```python
from build123d import *

# Parameters (mm, degrees)
SKETCH_2_W          = 51.075539497
SKETCH_2_H          = 30.123383878
CUT_EXTRUDE_1_DEPTH = 40
SKETCH_3_W          = 2.341501377
SKETCH_3_H          = 8.048910983
SKETCH_3_W_2        = 1.756126033
SKETCH_3_H_2        = 6.841574336
CUT_EXTRUDE_2_DEPTH = 20


with BuildPart() as part:
    # Эскиз1 → Повернуть1 (revolve)
    with BuildSketch(Plane.XY, mode=Mode.PRIVATE) as revolve_1_sk:
        Polygon((-9.75, 20), (-8.75, 20), (-8.75, 11), (8.75, 11), (8.75, 20), (9.75, 20), (9.75, 10), (-9.75, 10), align=None)
    revolve(revolve_1_sk.sketch.rotate(Axis((-17.336723769, 0, 0), (1, 0, 0)), 90), axis=Axis((-17.336723769, 0, 0), (1, 0, 0)))

    # Эскиз2 → Вырез-Вытянуть1 (cut)
    with BuildSketch(Plane(origin=(9.75, 0, 0), x_dir=(0, 0, -1), z_dir=(1, 0, 0))):
        with Locations((-1.37941238, -13.061691939)):
            Rectangle(SKETCH_2_W, SKETCH_2_H)
    extrude(amount=-CUT_EXTRUDE_1_DEPTH, mode=Mode.SUBTRACT)

    # Эскиз3 → Вырез-Вытянуть2 (cut)
    with BuildSketch(Plane(origin=(9.75, 0, 0), x_dir=(0, 0, -1), z_dir=(1, 0, 0))):
        with Locations((-20.670750689, 2.548643467)):
            Rectangle(SKETCH_3_W, SKETCH_3_H)
        with Locations((20.378063017, 2.310834734)):
            Rectangle(SKETCH_3_W_2, SKETCH_3_H_2)
    extrude(amount=-CUT_EXTRUDE_2_DEPTH, mode=Mode.SUBTRACT)


solid = part.part
```
Read the model definition and answer for the solid it produces. Units are mm, in the model's axes. A direction names the side the tool comes from. Give positions to 0.01 mm unless a question says otherwise; leave off trailing zeros. Order: outer loops, then holes, each group sorted by start corner. A loop starts at its lowest first (then second) coordinate and runs counter-clockwise, first axis right, second up. Notation, with made-up numbers: (-36, 6.5) -> (-23, 6.5) arc R24 cw to (-23, 17.5) -> close; hole circle Ø5 at (31.5, -28.75). An arc over 180 degrees is marked (long way). Write item = value, one per line.
1. A cutting plane is placed at B-B, the plane z = 14. Write down the section's boundary in (x, y), and give its area (3 significant figures).
Numbers:
outline = (-9.75, 2) -> (-8.75, 2) -> (-8.75, 14.28) -> (-9.75, 14.28) -> close; (8.75, 2) -> (9.75, 2) -> (9.75, 14.28) -> (8.75, 14.28) -> close
area = 24.6 mm²
2. A cutting plane is placed at A-A, the plane y = 12. Write down the section's boundary in (x, z).
Numbers:
outline = (-9.75, -16) -> (-8.75, -16) -> (-8.75, 16) -> (-9.75, 16) -> close; (8.75, -16) -> (9.75, -16) -> (9.75, 16) -> (8.75, 16) -> close
3. The mould has two halves that part along X. Classify faces 1 (the face through (0, 11, 0)), 2 (the face through (9.75, 11, 0)), 3 (the face through (9, 3, 19.5)), 4 (the face through (-9.75, 11, 0)): +X half, -X half, draft (parallel to the pull), parting line (faces both ways), or undercut.
Numbers:
face_1 = undercut
face_2 = +X half
face_3 = draft
face_4 = -X half
4. For faces 5 (the face through (-9, 3, 19.5)), 6 (the face through (8.75, 13, 0)), determine the directions among +Z, -Z, +X, -X, +Y, -Y from which every point of the face is accessible in a straight line to the end or side of a thin tool.
Numbers:
face_5 = +Z, +X, -X, +Y, -Y
face_6 = +Y
5. Given pin 1 (1.5 mm diameter, centred on x = -1.5, z = 4, fed in from -Y); pin 2 (2 mm diameter, centred on x = -7, z = 3.5, fed in from +Y); pin 3 (8 mm diameter, centred on x = 4, z = -4, fed in from -Y), each flat-ended and moving along its own axis, determine where each tip first touches the part or whether it passes through.
Numbers:
pin_1 = 8.8
pin_2 = 10.71
pin_3 = 6
6. Straight lines are drawn through the part: line 1 along X through (y, z) = (14, 5); line 2 along Z through (x, y) = (5.5, 8.5); line 3 along Z through (x, y) = (-1.25, 4). For each, find the intervals that lie inside material, in ascending order.
Numbers:
line_1 = -9.75 to -8.75, 8.75 to 9.75
line_2 = -6.98 to -5.27, 5.27 to 6.98
line_3 = -10.25 to -9.17, 9.17 to 10.25
7. A cutting plane is placed at D-D, the plane z = 8. Write down the section's boundary in (x, y), and give its area (3 significant figures).
Numbers:
outline = (-9.75, 6) -> (9.75, 6) -> (9.75, 18.33) -> (8.75, 18.33) -> (8.75, 7.55) -> (-8.75, 7.55) -> (-8.75, 18.33) -> (-9.75, 18.33) -> close
area = 51.8 mm²
8. A cutting plane is placed at C-C, the plane x = -1.5. Write down the section's boundary in (y, z).
Numbers:
outline = (2, -10.82) arc R11 ccw to (2, 10.82) -> (2, 9.8) arc R10 cw to (2, -9.8) -> close
